from build123d import *

# Parameters (mm, degrees)
SKETCH_2_W          = 18.8
SKETCH_2_H          = 22.1
EXTRUDE_1_DEPTH     = 64.2
SKETCH_4_R          = 3.6
EXTRUDE_2_DEPTH     = 0.1
SKETCH_5_R          = 2.7
EXTRUDE_3_DEPTH     = 9.1
CUT_EXTRUDE_START   = -7.9
CUT_EXTRUDE_1_DEPTH = 7.9
CUT_EXTRUDE_2_DEPTH = 27
CUT_EXTRUDE_3_DEPTH = 10
FILLET_1_R          = 2
SKETCH_10_R         = 1.5
CUT_EXTRUDE_4_DEPTH = 3


with BuildPart() as part:
    # 草图2 → 凸台-拉伸1 (new body)
    with BuildSketch(Plane(origin=(0, 0, 0), x_dir=(0, 0, -1), z_dir=(1, 0, 0))):
        Rectangle(SKETCH_2_W, SKETCH_2_H)
    extrude(amount=EXTRUDE_1_DEPTH)

    # 草图4 → 凸台-拉伸2 (add)
    with BuildSketch(Plane.XY.offset(9.4)):
        with Locations(Location((11.2, 0, 0), (0, 0, 180))):
            Circle(SKETCH_4_R)
    extrude(amount=EXTRUDE_2_DEPTH)

    # 草图5 → 凸台-拉伸3 (add)
    with BuildSketch(Plane.XY.offset(9.4)):
        with Locations(Location((11.2, 0, 0), (0, 0, 180))):
            Circle(SKETCH_5_R)
    extrude(amount=EXTRUDE_3_DEPTH)

    # 草图6 → 切除-拉伸1 (cut)
    with BuildSketch(Plane.XY.offset(18.5).offset(CUT_EXTRUDE_START)):
        with BuildLine():
            Line((9.35, -1.966596044), (9.35, 1.966596044))
            ThreePointArc((9.35, 1.966596044), (8.5, 0), (9.35, -1.966596044))
        make_face()
        with BuildLine():
            ThreePointArc((13.9, 0), (13.678406746, 1.071214264), (13.05, 1.966596044))
            Line((13.05, 1.966596044), (13.05, -1.966596044))
            ThreePointArc((13.05, -1.966596044), (13.678406746, -1.071214264), (13.9, 0))
        make_face()
    extrude(amount=CUT_EXTRUDE_1_DEPTH, mode=Mode.SUBTRACT)

    # 草图7 → 切除-拉伸2 (cut)
    with BuildSketch(Plane(origin=(64.2, 0, 0), x_dir=(0, 0, -1), z_dir=(1, 0, 0))):
        with BuildLine():
            ThreePointArc((-9.4, 6.180817098), (-6.249642407, 9.354382384), (-2.111871208, 11.05))
            Line((-2.111871208, 11.05), (-9.4, 11.05))
            Line((-9.4, 11.05), (-9.4, 6.180817098))
        make_face()
        with BuildLine():
            ThreePointArc((2.111871208, 11.05), (6.249642407, 9.354382384), (9.4, 6.180817098))
            Line((9.4, 6.180817098), (9.4, 11.05))
            Line((9.4, 11.05), (2.111871208, 11.05))
        make_face()
        with BuildLine():
            Line((2.111871208, -11.05), (9.4, -11.05))
            Line((9.4, -11.05), (9.4, -6.180817098))
            ThreePointArc((9.4, -6.180817098), (6.249642407, -9.354382384), (2.111871208, -11.05))
        make_face()
        with BuildLine():
            Line((-9.4, -11.05), (-2.111871208, -11.05))
            ThreePointArc((-2.111871208, -11.05), (-6.249642407, -9.354382384), (-9.4, -6.180817098))
            Line((-9.4, -6.180817098), (-9.4, -11.05))
        make_face()
    extrude(amount=-CUT_EXTRUDE_2_DEPTH, mode=Mode.SUBTRACT)

    # 草图9 → 切除-拉伸3 (cut)
    with BuildSketch(Plane(origin=(64.2, 0, 0), x_dir=(0, 0, -1), z_dir=(1, 0, 0))):
        with BuildLine():
            Line((-9.4, 6.180817098), (-9.4, 3.411744422))
            ThreePointArc((-9.4, 3.411744422), (0, 10), (9.4, 3.411744422))
            Line((9.4, 3.411744422), (9.4, 6.180817098))
            ThreePointArc((9.4, 6.180817098), (6.249642407, 9.354382384), (2.111871208, 11.05))
            Line((2.111871208, 11.05), (-2.111871208, 11.05))
            ThreePointArc((-2.111871208, 11.05), (-6.249642407, 9.354382384), (-9.4, 6.180817098))
        make_face()
        with BuildLine():
            ThreePointArc((-9.4, -6.180817098), (-6.249642407, -9.354382384), (-2.111871208, -11.05))
            Line((-2.111871208, -11.05), (2.111871208, -11.05))
            ThreePointArc((2.111871208, -11.05), (6.249642407, -9.354382384), (9.4, -6.180817098))
            Line((9.4, -6.180817098), (9.4, -3.411744422))
            ThreePointArc((9.4, -3.411744422), (0, -10), (-9.4, -3.411744422))
            Line((-9.4, -3.411744422), (-9.4, -6.180817098))
        make_face()
    extrude(amount=-CUT_EXTRUDE_3_DEPTH, mode=Mode.SUBTRACT)

    # 圆角1
    # the kernel refuses this fillet: 2 mm, written as the material it takes off along each edge
    with BuildSketch(Plane(origin=(64.2, 0, 0), x_dir=(0, -0.15173257370011314, 0.9884215831710372), z_dir=(0, -0.9884215831710372, -0.15173257370011314))) as fillet_1_piece_1:
        with BuildLine():
            CenterArc((10 - FILLET_1_R, FILLET_1_R), FILLET_1_R, 270, 90)
            Line((10 - FILLET_1_R, 0), (10, 0))
            Line((10, 0), (10, FILLET_1_R))
        make_face()
    revolve(axis=Axis((64.2, 0, 0), (-1, 0, 0)), revolution_arc=197.454690212, mode=Mode.SUBTRACT)
    with BuildSketch(Plane(origin=(64.2, 0, 0), x_dir=(0, 0.1517325737001477, -0.9884215831710319), z_dir=(0, 0.9884215831710319, 0.1517325737001477))) as fillet_1_piece_2:
        with BuildLine():
            CenterArc((10 - FILLET_1_R, FILLET_1_R), FILLET_1_R, 270, 90)
            Line((10, FILLET_1_R), (10, 0))
            Line((10, 0), (10 - FILLET_1_R, 0))
        make_face()
    revolve(axis=Axis((64.2, 0, 0), (-1, 0, 0)), revolution_arc=197.454690212, mode=Mode.SUBTRACT)

    # 草图10 → 切除-拉伸4 (cut)
    with BuildSketch(Plane.XY.offset(9.4)):
        with Locations((31.8, 8.75)):
            Circle(SKETCH_10_R)
        with Locations(Location((31.8, -8.75, 0), (0, 0, 180))):
            Circle(SKETCH_10_R)
    extrude(amount=-CUT_EXTRUDE_4_DEPTH, mode=Mode.SUBTRACT)


solid = part.part
Input: part model. Units: mm. Frame: model coordinates. A direction names the side the tool comes from. Give positions to 0.01 mm unless a question says otherwise; leave off trailing zeros. Write each loop counter-clockwise with the first axis right and the second up, starting at its lowest first coordinate (ties: lowest second). Pieces come first, ordered by that corner, then holes.
Q1. Section A-A, the plane x = 53.5. Output: boundary loops of the cut face in (y, z), plus the area to 3 significant figures.
Q2. Section C-C, the plane x = 31.8. Output: boundary loops of the cut face in (y, z), plus the area to 3 significant figures.
Q3. Section D-D, the plane x = 11.2. Output: boundary loops of the cut face in (y, z), plus the area to 3 significant figures.
Q4. Material intervals for probe 1 along Y at (x, z) = (31.8, 7.4); probe 2 along X at (y, z) = (-8.75, 8.7); probe 3 along X at (y, z) = (8.5, -6), sorted ascending.
Q5. First-contact query: P1, Ø1, axis at x = 40, y = -4.5, coming from the +Z side; P2, Ø2.5, axis at x = 31.8, y = -8.75, coming from the +Z side; P3, Ø1, axis at x = 57, y = 9, coming from the +Z side. Flat tips, straight axial feed; report the tip coordinate or a pass-through.
Q6. Set-up query: faces 1 (the face through (37.2, -10, -7)), 2 (the face through (11, -3, 9.5)), 3 (the face through (54.2, 10.4, 0.7)), 4 (the face through (54.2, -10.3, 0)). Return all of +Z, -Z, +X, -X, +Y, -Y with unobstructed straight access to the full face (end or side cutting, diameter ignored); none if empty.
Q7. Section B-B, the plane y = 0. Output: boundary loops of the cut face in (x, z), plus the area to 3 significant figures.
Q8. Pull-direction query (X, two-part tool) for faces 5 (the face through (32, -9, 6.4)), 6 (the face through (32.125, -7.286, 7.921)), 7 (the face through (64.2, 0, 0)), 8 (the face through (45.819, 9.389, -6.197)); classes: pulls with the +X half, pulls with the -X half, needs draft (parallel to the pull), parting line crosses it, or undercut.
Filled in:
1. outline: (-11.05, -2.11) arc R11.25 ccw to (-6.18, -9.4) - (6.18, -9.4) arc R11.25 ccw to (11.05, -2.11) - (11.05, 2.11) arc R11.25 ccw to (6.18, 9.4) - (-6.18, 9.4) arc R11.25 ccw to (-11.05, 2.11) - close
1. area: 365 mm2
2. outline: (-11.05, -9.4) - (11.05, -9.4) - (11.05, 9.4) - (10.25, 9.4) - (10.25, 6.4) - (7.25, 6.4) - (7.25, 9.4) - (-7.25, 9.4) - (-7.25, 6.4) - (-10.25, 6.4) - (-10.25, 9.4) - (-11.05, 9.4) - close
2. area: 397 mm2
3. outline: (-11.05, -9.4) - (11.05, -9.4) - (11.05, 9.4) - (3.6, 9.4) - (3.6, 9.5) - (2.7, 9.5) - (2.7, 18.5) - (-2.7, 18.5) - (-2.7, 9.5) - (-3.6, 9.5) - (-3.6, 9.4) - (-11.05, 9.4) - close
3. area: 465 mm2
4. probe 1: y = -11.05 to -10.25, -7.25 to 7.25, 10.25 to 11.05
4. probe 2: x = 0 to 30.3, 33.3 to 37.2
4. probe 3: x = 0 to 54.2
5. P1: stops at z = 9.4
5. P2: stops at z = 6.4
5. P3: stops at z = 5.27
6. face 1: -Z, +X, -Y
6. face 2: +Z
6. face 3: +X, +Y
6. face 4: +X, -Y
7. outline: (0, -9.4) - (63.63, -9.4) arc R2 ccw to (64.2, -8) - (64.2, 8) arc R2 ccw to (63.63, 9.4) - (14.8, 9.4) - (14.8, 9.5) - (13.9, 9.5) - (13.9, 10.6) - (13.05, 10.6) - (13.05, 18.5) - (9.35, 18.5) - (9.35, 10.6) - (8.5, 10.6) - (8.5, 9.5) - (7.6, 9.5) - (7.6, 9.4) - (0, 9.4) - close
7. area: 1,240 mm2
8. face 5: undercut
8. face 6: undercut
8. face 7: pulls with the +X half
8. face 8: needs draft
